from build123d import *

# Parameters (mm, degrees)
CUT_EXTRUDE1_START = -96
CUT_EXTRUDE1_DEPTH = 96


with BuildPart() as part:
    # Sketch2 → Revolve1 (revolve)
    with BuildSketch(Plane.XY, mode=Mode.PRIVATE) as revolve1_sk:
        with BuildLine():
            Line((10, 64), (-10, 64))
            ThreePointArc((-10, 64), (-17.071067812, 61.071067812), (-20, 54))
            Line((-20, 54), (-20, 41.275))
            Line((-20, 41.275), (-30, 31.795))
            Line((-30, 31.795), (-30, 16.795))
            Line((-30, 16.795), (-31.5875, 16.795))
            Line((-31.5875, 16.795), (-31.5875, 7.25))
            Line((-31.5875, 7.25), (-34, 7.25))
            Line((-34, 7.25), (-34, 6))
            Line((-34, 6), (-48, 6))
            Line((-48, 6), (-48, 0))
            Line((-48, 0), (48, 0))
            Line((48, 0), (48, 6))
            Line((48, 6), (34, 6))
            Line((34, 6), (34, 7.25))
            Line((34, 7.25), (31.5875, 7.25))
            Line((31.5875, 7.25), (31.5875, 16.795))
            Line((31.5875, 16.795), (30, 16.795))
            Line((30, 16.795), (30, 31.795))
            Line((30, 31.795), (20, 41.275))
            Line((20, 41.275), (20, 54))
            ThreePointArc((20, 54), (17.071067812, 61.071067812), (10, 64))
        make_face()
    revolve(revolve1_sk.sketch.rotate(Axis((-48, 0, 0), (1, 0, 0)), 90), axis=Axis((-48, 0, 0), (1, 0, 0)))

    # Sketch3 → Cut-Extrude1 (cut)
    with BuildSketch(Plane.ZY.offset(48).offset(CUT_EXTRUDE1_START)):
        with BuildLine():
            Line((5, 3.31662479), (5, -3.31662479))
            ThreePointArc((5, -3.31662479), (6, 0), (5, 3.31662479))
        make_face()
        with BuildLine():
            Line((-5, 3.31662479), (-5, -3.31662479))
            ThreePointArc((-5, -3.31662479), (-6, 0), (-5, 3.31662479))
        make_face()
    cut_extrude1 = extrude(amount=CUT_EXTRUDE1_DEPTH, mode=Mode.SUBTRACT)

    # Mirror1: Cut-Extrude1 across plane
    add(cut_extrude1.mirror(Plane(origin=(0, 0, 0), x_dir=(0, 0, 1), z_dir=(1, 0, 0))), mode=Mode.SUBTRACT)


solid = part.part
Work out the finished part from the listing and answer in its coordinate system (mm). A direction names the side the tool comes from. Round coordinates to 2 decimals unless told otherwise and drop trailing zeros. Write each loop counter-clockwise with the first axis right and the second up, starting at its lowest first coordinate (ties: lowest second). Pieces come first, ordered by that corner, then holes. Notation, with made-up numbers: (16.5, 25.5) - (44.5, 25.5) arc R22 ccw to (44.5, 53.5) - close; hole circle Ø11 at (34, 44.25). An arc over 180 degrees is marked (long way). Answer in a Markdown table with one row per item. Add a question column.
1. The mould has two halves that part along Y. Classify faces 1 (the cylindrical face through (0, 0, -6)), 2 (the conical face through (29.374, -9.728, 30.892)), 3 (the flat face through (-20, 40, -12)): +Y half, -Y half, draft (parallel to the pull), parting line (faces both ways), or undercut.
2. Find the intervals of material crossed by line 1 along X through (y, z) = (4, -29); line 2 along X through (y, z) = (0.5, 6.5); line 3 along Z through (x, y) = (33, 3), in increasing order. Write a range as from..to.
3. A cutting plane is placed at A-A, the plane x = 26.5. Determine the outline of the cut face in (y, z), and give its area (3 significant figures).
4. For faces 4 (the cylindrical face through (-41, -6, 0)), 5 (the cylindrical face through (32.78, 6.43, 3.35)), 6 (the flat face through (-30, 14, 14)), 7 (the cylindrical face through (41, -6, 0)), determine the directions among +Z, -Z, +X, -X, +Y, -Y from which every point of the face is accessible in a straight line to the end or side of a thin tool.
5. Given pin 1 (12 mm diameter, centred on x = 8.5, z = 40.5, fed in from +Y) (3 decimals); pin 2 (4 mm diameter, centred on x = -3, z = -36.5, fed in from -Y) (3 decimals); pin 3 (5 mm diameter, centred on x = 0, z = 33, fed in from +Y) (3 decimals), each flat-ended and moving along its own axis, determine where each tip first touches the part or whether it passes through.
6. A cutting plane is placed at B-B, the plane y = 0. Count the separate pieces of the cut face and the enclosed holes in it, and give its area (3 significant figures).
Worked out:
| question | item | result |
|---|---|---|
| 1 | face 1 | undercut |
| 1 | face 2 | parting line |
| 1 | face 3 | draft |
| 2 | line 1 | -30..30 |
| 2 | line 2 | -34..34 |
| 2 | line 3 | -6.6..-5.2, -5..5, 5.2..6.6 |
| 3 | outline | circle Ø70.23 at (0, 0); hole (-3.32, -5) arc R6 ccw to (3.32, -5) - close; hole (-3.32, 5) - (3.32, 5) arc R6 ccw to start |
| 3 | area | 3,860 mm^2 |
| 4 | face 4 | -X, -Y |
| 4 | face 5 | +X |
| 4 | face 6 | -X |
| 4 | face 7 | +X, -Y |
| 5 | pin 1 | y = 53.905 |
| 5 | pin 2 | y = -53.905 |
| 5 | pin 3 | y = 56.265 |
| 6 | separate pieces | 3 |
| 6 | enclosed holes | 0 |
| 6 | area | 6,820 mm^2 |
